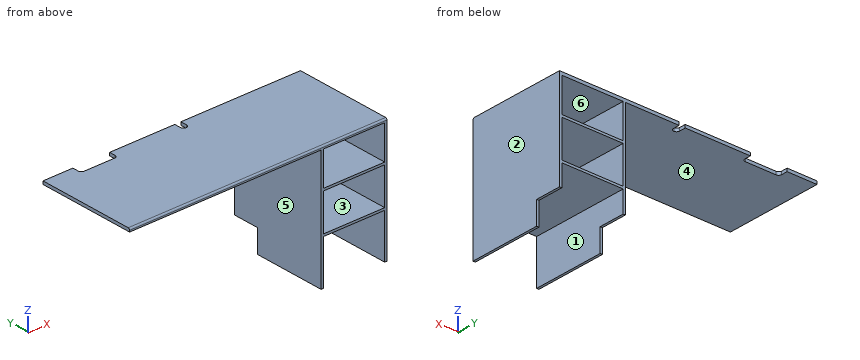
from build123d import *

# Parameters (mm, degrees)
F1_DEPTH      = 25.4
F2_R          = 12.7
F3_W          = 508
F3_H          = 19.05
F4_DEPTH      = 406.4
F4_DEPTH_BACK = 406.4
F5_W          = 215.9
F5_H          = 190.5
F6_DEPTH      = 2133.601


with BuildPart() as f1:
    # F0 (on Top) → F1 (new body)
    with BuildSketch(Plane.XY):
        with BuildLine():
            Line((-819.15, 406.4), (-1066.8, 406.4))
            Line((-1066.8, 406.4), (-1066.8, -406.4))
            Line((-1066.8, -406.4), (1066.8, -406.4))
            Line((1066.8, -406.4), (1066.8, 406.4))
            Line((1066.8, 406.4), (76.2, 406.4))
            Line((76.2, 406.4), (76.2, 353.484618))
            ThreePointArc((76.2, 353.484618), (68.760512, 335.524106), (50.8, 328.084618))
            ThreePointArc((50.8, 328.084618), (32.839488, 335.524106), (25.4, 353.484618))
            Line((25.4, 353.484618), (25.4, 406.4))
            Line((25.4, 406.4), (-514.35, 406.4))
            Line((-514.35, 406.4), (-514.35, 355.6))
            ThreePointArc((-514.35, 355.6), (-521.789488, 337.639488), (-539.75, 330.2))
            Line((-539.75, 330.2), (-793.75, 330.2))
            ThreePointArc((-793.75, 330.2), (-811.710512, 337.639488), (-819.15, 355.6))
            Line((-819.15, 355.6), (-819.15, 406.4))
        make_face()
    extrude(amount=F1_DEPTH)

    # F2
    f2_edges = [f1.edges().sort_by_distance(p)[0] for p in [
        (0, -406.4, 25.4),
    ]]
    fillet(f2_edges, radius=F2_R)

    # F3 (on Front) → F4 (join, two sides)
    with BuildSketch(Plane.XZ) as f4_sk:
        Polygon((1066.8, -990.6), (1066.8, 0), (1047.75, 0), (1047.75, -279.4), (1047.75, -298.45), (1047.75, -603.25), (1047.75, -622.3), (1047.75, -990.6), align=None)
        Polygon((539.75, -298.45), (539.75, -279.4), (539.75, 0), (520.7, 0), (520.7, -990.6), (539.75, -990.6), (539.75, -622.3), (539.75, -603.25), align=None)
        with Locations((793.75, -288.925)):
            Rectangle(F3_W, F3_H)
        with Locations((793.75, -612.775)):
            Rectangle(F3_W, F3_H)
    extrude(amount=F4_DEPTH)
    extrude(f4_sk.sketch, amount=-F4_DEPTH_BACK)

    # F5 (on face) → F6 (cut, through all)
    with BuildSketch(Plane.YZ.offset(1066.8)):
        with Locations((298.45, -895.35)):
            Rectangle(F5_W, F5_H)
    extrude(amount=-F6_DEPTH, mode=Mode.SUBTRACT)


solid = f1.part
Input: part model. Units: mm. Frame: model coordinates. Face numbers are marked on the shaded views. A direction names the side the tool comes from. Coordinates: 2 decimals unless noted, no trailing zeros. Loops run counter-clockwise (first coordinate to the right, second up) from the corner with the lowest first, then second, coordinate; pieces in that order, holes last.
(1) Pull-direction query (X, two-part tool) for the marked faces 4, 5 and 6; classes: released by +X, released by -X, zero draft, split by the parting line, or undercut.
(2) Section B-B on z = -849. Return the cut outline in (x, y), then the cut area to 3 significant figures.
(3) Set-up query: the marked faces 1, 2 and 3. Return all of +Z, -Z, +X, -X, +Y, -Y with unobstructed straight access to the full face (end or side cutting, diameter ignored); none if empty.
(4) Material intervals for probe 1 along Z at (x, y) = (908, -361); probe 2 along X at (y, z) = (-161, -213); probe 3 along Z at (x, y) = (54.5, -325.5), sorted ascending.
(5) Section A-A on x = 932. Return the cut outline in (y, z).
(6) First-contact query: pin 1 Ø15 at (x, z) = (1058, -892) entering from +Y; pin 2 Ø1 at (x, y) = (-316.5, -96.5) entering from -Z; pin 3 Ø7.5 at (x, z) = (-729.5, 6.5) entering from +Y. Flat tips, straight axial feed; report the tip coordinate or a pass-through.
(7) Section C-C on y = 25. Return the cut outline in (x, z).
(8) Section D-D on x = 263. Return the cut outline in (y, z), then the cut area to 3 significant figures.
Data:
1. face 4: zero draft
1. face 5: released by -X
1. face 6: undercut
2. outline: (520.7, -406.4) - (539.75, -406.4) - (539.75, 190.5) - (520.7, 190.5) - close; (1047.75, -406.4) - (1066.8, -406.4) - (1066.8, 190.5) - (1047.75, 190.5) - close
2. area: 22,700 mm2
3. face 1: -Z, +Y, -Y
3. face 2: +Z, -Z, +X, +Y, -Y
3. face 3: +Y, -Y
4. probe 1: z = -622.3 to -603.25, -298.45 to -279.4, 0 to 25.4
4. probe 2: x = 520.7 to 539.75, 1047.75 to 1066.8
4. probe 3: z = 0 to 25.4
5. outline: (-406.4, -622.3) - (406.4, -622.3) - (406.4, -603.25) - (-406.4, -603.25) - close; (-406.4, -298.45) - (406.4, -298.45) - (406.4, -279.4) - (-406.4, -279.4) - close; (-406.4, 0) - (406.4, 0) - (406.4, 25.4) - (-393.7, 25.4) arc R12.7 ccw to (-406.4, 12.7) - close
6. pin 1: stops at y = 190.5
6. pin 2: stops at z = 0
6. pin 3: stops at y = 330.2
7. outline: (-1066.8, 0) - (520.7, 0) - (520.7, -990.6) - (539.75, -990.6) - (539.75, -622.3) - (1047.75, -622.3) - (1047.75, -990.6) - (1066.8, -990.6) - (1066.8, 25.4) - (-1066.8, 25.4) - close; hole (539.75, -603.25) - (1047.75, -603.25) - (1047.75, -298.45) - (539.75, -298.45) - close; hole (539.75, -279.4) - (1047.75, -279.4) - (1047.75, 0) - (539.75, 0) - close
8. outline: (-406.4, 0) - (406.4, 0) - (406.4, 25.4) - (-393.7, 25.4) arc R12.7 ccw to (-406.4, 12.7) - close
8. area: 20,600 mm2
